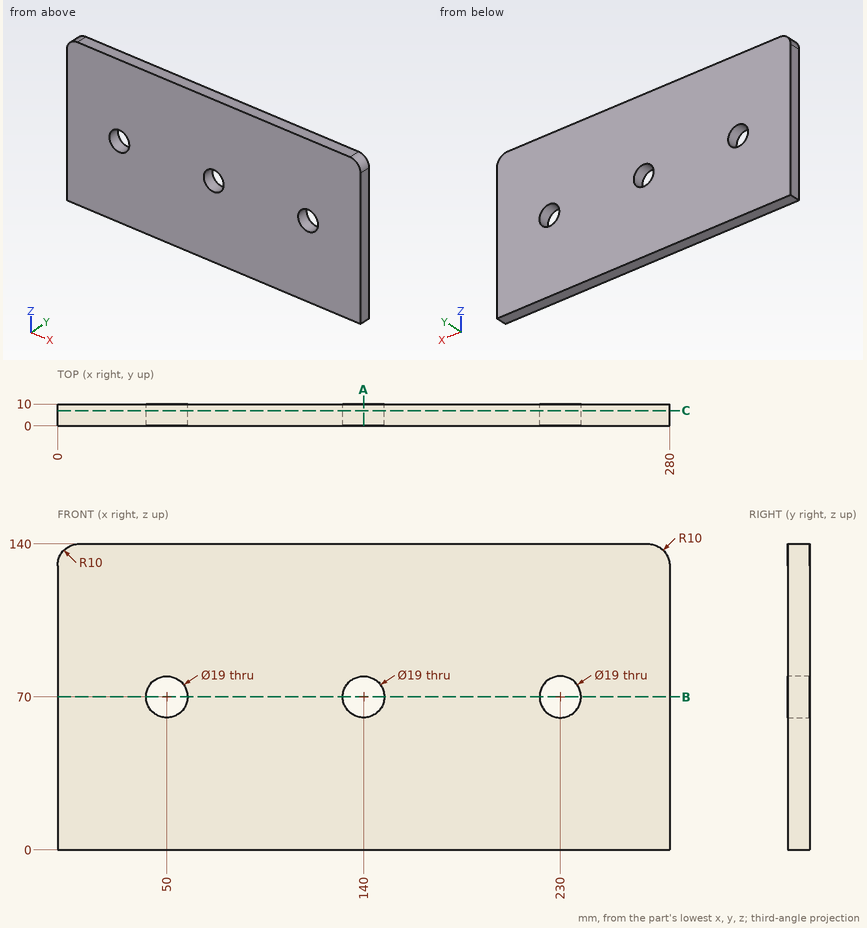
Verification items for this drawing (mm, ordinates from the low corner). Coordinates: 2 decimals unless noted, no trailing zeros. Write each loop counter-clockwise with the first axis right and the second up, starting at its lowest first coordinate (ties: lowest second). Pieces come first, ordered by that corner, then holes. Notation, with made-up numbers: M 73.5,11.25 L 84.5,11.25 A7 cw 84.5,20.25 Z; hole C 73.25,28 d5. An arc over 180 degrees is marked long. Answer as a JSON object with one key per item and string values. Group by question number.
(1) Cross-section at C-C, the plane y = 7. Record the cut outline in (x, z), and give its area (3 significant figures).
(2) Cross-section at B-B, the plane z = 70. Record the cut outline in (x, y).
(3) Material ranges on line 1 (X direction, y = 6.5, z = 70); line 2 (Z direction, x = 230, y = 4); line 3 (X direction, y = 6.75, z = 71.5), recorded low to high.
(4) Gauge pin test, flat ends, axial feed: pin 1 (1.5 mm diameter, centred on x = 95.5, y = 6.5, fed in from -Z); pin 2 (11.5 mm diameter, centred on x = 140, z = 70, fed in from -Y). Record the tip position at first contact, or that the pin passes through.
(5) Cross-section at A-A, the plane x = 140. Record the cut outline in (y, z), and give its area (3 significant figures).
Reply:
{
 "1": {"outline": "M 0,0 L 280,0 L 280,130 A10 ccw 270,140 L 10,140 A10 ccw 0,130 Z; hole C 50,70 d19; hole C 140,70 d19; hole C 230,70 d19", "area": "38,300 mm²"},
 "2": {"outline": "M 0,0 L 40.5,0 L 40.5,10 L 0,10 Z; M 59.5,0 L 130.5,0 L 130.5,10 L 59.5,10 Z; M 149.5,0 L 220.5,0 L 220.5,10 L 149.5,10 Z; M 239.5,0 L 280,0 L 280,10 L 239.5,10 Z"},
 "3": {"line 1": "0 to 40.5, 59.5 to 130.5, 149.5 to 220.5, 239.5 to 280", "line 2": "0 to 60.5, 79.5 to 140", "line 3": "0 to 40.62, 59.38 to 130.62, 149.38 to 220.62, 239.38 to 280"},
 "4": {"pin 1": "z = 0", "pin 2": "through"},
 "5": {"outline": "M 0,0 L 10,0 L 10,60.5 L 0,60.5 Z; M 0,79.5 L 10,79.5 L 10,140 L 0,140 Z", "area": "1,210 mm²"}
}
